Can you work these out from the model? Positions are in its coordinate system, mm. A direction names the side the tool comes from. Give positions to 0.01 mm unless a question says otherwise; leave off trailing zeros. Order: outer loops, then holes, each group sorted by start corner. A loop starts at its lowest first (then second) coordinate and runs counter-clockwise, first axis right, second up. Notation, with made-up numbers: (8, -12) - (49, -12) arc R31 ccw to (49, 18) - close; hole circle Ø9 at (-2, 4.5). An arc over 180 degrees is marked (long way). Use one line per item in the form item = value. Start each with the question number.
1) Suppose I cut it at A-A, the plane z = 21.5. Write out the boundary of the cut face in (x, y).
2) Suppose I cut it at C-C, the plane z = 7.5. Write out the boundary of the cut face in (x, y).
3) Suppose I cut it at D-D, the plane x = -61. Write out the boundary of the cut face in (y, z), and give its area (3 significant figures).
4) Please list where these lines run through material, in increasing order: probe 1 along X at (y, z) = (-2.5, -7.5); probe 2 along Z at (x, y) = (-20.19, 1.75); probe 3 along X at (y, z) = (5, -21.5).
5) Suppose I cut it at B-B, the plane x = -34.5. Write out the boundary of the cut face in (y, z).
6) We'd pull the mould along Z, two halves only. Please class faces 1 (the cylindrical face through (-67.646, -0.063, 15.796)), 2 (the cylindrical face through (-15.641, -0.063, -31.297)), 3 (the cylindrical face through (-79.513, -0.063, -7.305)): released by +Z, released by -Z, zero draft, split by the parting line, or undercut.
7) Which directions (+Z, -Z, +X, -X, +Y, -Y) give clear straight access to the entire face, cutting with the end or side of a thin tool? Please do faces 4 (the flat face through (-75, 0, -15.5)), 5 (the flat face through (-75, 0, 15.5)), 6 (the flat face through (-30, -2, -10)).
8) For pin 1 (2 mm diameter, centred on x = -65, y = 0, fed in from +Z); pin 2 (1.5 mm diameter, centred on y = -3, z = 3, fed in from +X); pin 3 (4 mm diameter, centred on x = -59.5, z = 0.5, fed in from +Y); pin 4 (1.8 mm diameter, centred on x = -61, z = -7.5, fed in from -Y), each with a flat end and sliding along its axis, tell me the tip position at first contact or that it passes through.
```python
from build123d import *

# Parameters (mm, degrees)
SKETCH1_R               = 12
BOSS_EXTRUDE1_DEPTH     = 4.5
SKETCH2_R               = 1.7
CUT_EXTRUDE1_DEPTH      = 91.980767198
FILLET1_R               = 4
CUT_EXTRUDE4_DEPTH      = 91.980767198
SKETCH6_R               = 1.5
CUT_EXTRUDE5_DEPTH      = 41
CUT_EXTRUDE6_START      = -6
SKETCH7_W               = 30
SKETCH7_H               = 20
CUT_EXTRUDE6_DEPTH      = 3
SKETCH8_W               = 30
SKETCH8_H               = 17
CUT_EXTRUDE7_DEPTH      = 9
FILLET5_R               = 4
SKETCH10_W              = 10
SKETCH10_H              = 22.5
BOSS_EXTRUDE2_DEPTH     = 9
SKETCH13_R              = 3
BOSS_EXTRUDE4_DEPTH     = 2
CUT_EXTRUDE8_DEPTH      = 5
CUT_EXTRUDE8_DEPTH_BACK = 9
SKETCH11_R              = 2
FILLET6_R               = 4
BOSS_EXTRUDE3_DEPTH     = 9
FILLET8_R               = 4
SKETCH14_R              = 2
CUT_EXTRUDE9_DEPTH      = 16


with BuildPart() as part:
    # Sketch1 → Boss-Extrude1 (new, symmetric)
    with BuildSketch(Plane(origin=(0, 0, 0), x_dir=(1, 0, 0), z_dir=(0, 1, 0))):
        Polygon((21.5, 20), (21.5, -20), (-20.5, -32.5), (-84.5, -32.5), (-84.5, 32.5), (-20.5, 32.5), align=None)
        with Locations(Location((0, 0, 0), (0, 0, 270))):
            Circle(SKETCH1_R, mode=Mode.SUBTRACT)
    extrude(amount=BOSS_EXTRUDE1_DEPTH, both=True)

    # Sketch2 → Cut-Extrude1 (cut, through all)
    with BuildSketch(Plane(origin=(0, 4.5, 0), x_dir=(1, 0, 0), z_dir=(0, 1, 0))):
        with Locations(Location((15.5, 15.5, 0), (0, 0, 270))):
            Circle(SKETCH2_R)
        with Locations(Location((-15.5, 15.5, 0), (0, 0, 270))):
            Circle(SKETCH2_R)
        with Locations(Location((-15.5, -15.5, 0), (0, 0, 270))):
            Circle(SKETCH2_R)
        with Locations(Location((15.5, -15.5, 0), (0, 0, 270))):
            Circle(SKETCH2_R)
        with Locations(Location((-19.5, 27.5, 0), (0, 0, 270))):
            Circle(SKETCH2_R)
        with Locations(Location((-19.5, -27.5, 0), (0, 0, 270))):
            Circle(SKETCH2_R)
    extrude(amount=-CUT_EXTRUDE1_DEPTH, mode=Mode.SUBTRACT)

    # Fillet1
    fillet1_edges = [part.edges().sort_by_distance(p)[0] for p in [
        (-20.5, 0, 32.5),
        (-84.5, 0, 32.5),
        (-84.5, 0, -32.5),
        (-20.5, 0, -32.5),
        (21.5, 0, -20),
        (21.5, 0, 20),
    ]]
    fillet(fillet1_edges, radius=FILLET1_R)

    # Sketch5 → Cut-Extrude4 (cut, through all)
    with BuildSketch(Plane(origin=(0, 4.5, 0), x_dir=(1, 0, 0), z_dir=(0, 1, 0))):
        Polygon((-24.5, 32.5), (-24.5, 10), (-24.5, -10), (-24.5, -32.5), (26.912022907, -32.5), (26.912022907, 32.5), align=None)
    extrude(amount=-CUT_EXTRUDE4_DEPTH, mode=Mode.SUBTRACT)

    # Sketch6 → Cut-Extrude5 (cut)
    with BuildSketch(Plane.XZ.offset(4.5)):
        with Locations(Location((-81, -7.5, 0), (0, 0, 270))):
            Circle(SKETCH6_R)
        with Locations(Location((-81, 7.5, 0), (0, 0, 270))):
            Circle(SKETCH6_R)
        with Locations(Location((-61, -7.5, 0), (0, 0, 270))):
            Circle(SKETCH6_R)
        with Locations(Location((-61, 7.5, 0), (0, 0, 270))):
            Circle(SKETCH6_R)
    extrude(amount=-CUT_EXTRUDE5_DEPTH, mode=Mode.SUBTRACT)

    # Sketch7 → Cut-Extrude6 (cut)
    with BuildSketch(Plane(origin=(0, 4.5, 0), x_dir=(1, 0, 0), z_dir=(0, 1, 0)).offset(CUT_EXTRUDE6_START)):
        with Locations((-39.5, 0)):
            Rectangle(SKETCH7_W, SKETCH7_H)
    extrude(amount=-CUT_EXTRUDE6_DEPTH, mode=Mode.SUBTRACT)

    # Sketch8 → Cut-Extrude7 (cut)
    with BuildSketch(Plane(origin=(0, 4.5, 0), x_dir=(1, 0, 0), z_dir=(0, 1, 0))):
        with Locations((-69.5, 24)):
            Rectangle(SKETCH8_W, SKETCH8_H)
        with Locations((-69.5, -24)):
            Rectangle(SKETCH8_W, SKETCH8_H)
    extrude(amount=-CUT_EXTRUDE7_DEPTH, mode=Mode.SUBTRACT)

    # Fillet5
    fillet5_edges = [part.edges().sort_by_distance(p)[0] for p in [
        (-84.5, 0, -15.5),
        (-54.5, 0, -32.5),
        (-84.5, 0, 15.5),
        (-54.5, 0, 32.5),
    ]]
    fillet(fillet5_edges, radius=FILLET5_R)

    # Sketch10 → Boss-Extrude2 (add)
    with BuildSketch(Plane(origin=(0, 4.5, 0), x_dir=(1, 0, 0), z_dir=(0, 1, 0))):
        with Locations((-19.5, -21.25)):
            Rectangle(SKETCH10_W, SKETCH10_H)
        with Locations((-19.5, 21.25)):
            Rectangle(SKETCH10_W, SKETCH10_H)
    extrude(amount=-BOSS_EXTRUDE2_DEPTH)

    # Sketch13 → Boss-Extrude4 (add)
    with BuildSketch(Plane(origin=(0, 4.5, 0), x_dir=(1, 0, 0), z_dir=(0, 1, 0))):
        with Locations(Location((-20.19, -21.5, 0), (0, 0, 90))):
            Circle(SKETCH13_R)
        with Locations(Location((-20.19, 21.5, 0), (0, 0, 90))):
            Circle(SKETCH13_R)
    extrude(amount=BOSS_EXTRUDE4_DEPTH)

    # Sketch11 → Cut-Extrude8 (cut, two sides: drawn at the far end of the back side and taken through both)
    with BuildSketch(Plane(origin=(0, 4.5, 0), x_dir=(1, 0, 0), z_dir=(0, 1, 0)).offset(-CUT_EXTRUDE8_DEPTH_BACK)):
        with Locations(Location((-20.19, -21.5, 0), (0, 0, 270))):
            Circle(SKETCH11_R)
        with Locations(Location((-20.19, 21.5, 0), (0, 0, 90))):
            Circle(SKETCH11_R)
    extrude(amount=CUT_EXTRUDE8_DEPTH + CUT_EXTRUDE8_DEPTH_BACK, mode=Mode.SUBTRACT)

    # Fillet6
    fillet6_edges = [part.edges().sort_by_distance(p)[0] for p in [
        (-14.5, 0, 32.5),
        (-14.5, 0, -32.5),
    ]]
    fillet(fillet6_edges, radius=FILLET6_R)

    # Sketch12 → Boss-Extrude3 (add)
    with BuildSketch(Plane(origin=(0, 4.5, 0), x_dir=(1, 0, 0), z_dir=(0, 1, 0))):
        Polygon((-54.5, 28.5), (-67.5, 15.5), (-54.5, 15.5), align=None)
        Polygon((-54.5, -28.5), (-67.5, -15.5), (-54.5, -15.5), align=None)
    extrude(amount=-BOSS_EXTRUDE3_DEPTH)

    # Fillet8
    fillet8_edges = [part.edges().sort_by_distance(p)[0] for p in [
        (-54.5, 0, -28.5),
        (-54.5, 0, 28.5),
        (-67.5, 0, -15.5),
        (-67.5, 0, 15.5),
    ]]
    fillet(fillet8_edges, radius=FILLET8_R)

    # Sketch14 → Cut-Extrude9 (cut)
    with BuildSketch(Plane.XZ.offset(1.5)):
        with Locations(Location((-48.5, 0, 0), (0, 0, 270))):
            Circle(SKETCH14_R)
        with Locations(Location((-34.5, 0, 0), (0, 0, 270))):
            Circle(SKETCH14_R)
    extrude(amount=-CUT_EXTRUDE9_DEPTH, mode=Mode.SUBTRACT)


solid = part.part
```
Result sheet:
q1.outline = (-61.5, -4.5) - (-22.19, -4.5) - (-22.19, 6.5) - (-23.19, 6.5) - (-23.19, 4.5) - (-61.5, 4.5) - close; (-18.19, -4.5) - (-14.5, -4.5) - (-14.5, 4.5) - (-17.19, 4.5) - (-17.19, 6.5) - (-18.19, 6.5) - close
q2.outline = (-84.5, -4.5) - (-82.5, -4.5) - (-82.5, 4.5) - (-84.5, 4.5) - close; (-79.5, -4.5) - (-62.5, -4.5) - (-62.5, 4.5) - (-79.5, 4.5) - close; (-59.5, -4.5) - (-54.5, -4.5) - (-54.5, -1.5) - (-24.5, -1.5) - (-24.5, 4.5) - (-59.5, 4.5) - close
q3.outline = (-4.5, -22) - (4.5, -22) - (4.5, -9) - (-4.5, -9) - close; (-4.5, -6) - (4.5, -6) - (4.5, 6) - (-4.5, 6) - close; (-4.5, 9) - (4.5, 9) - (4.5, 22) - (-4.5, 22) - close
q3.area = 342 mm²
q4.probe_1 = -84.5 to -82.5, -79.5 to -62.5, -59.5 to -54.5
q4.probe_2 = -32.5 to -23.5, -19.5 to -10, 10 to 19.5, 23.5 to 32.5
q4.probe_3 = -23.19 to -22.19, -18.19 to -17.19
q5.outline = (-4.5, -32.5) - (4.5, -32.5) - (4.5, -2) - (-1.5, -2) - (-1.5, -10) - (-4.5, -10) - close; (-4.5, 10) - (-1.5, 10) - (-1.5, 2) - (4.5, 2) - (4.5, 32.5) - (-4.5, 32.5) - close
q6.face_1 = released by +Z
q6.face_2 = released by -Z
q6.face_3 = undercut
q7.face_4 = -Z, -X, +Y, -Y
q7.face_5 = +Z, -X, +Y, -Y
q7.face_6 = +X, -Y
q8.pin_1 = 19
q8.pin_2 = -54.5
q8.pin_3 = 4.5
q8.pin_4 = through
